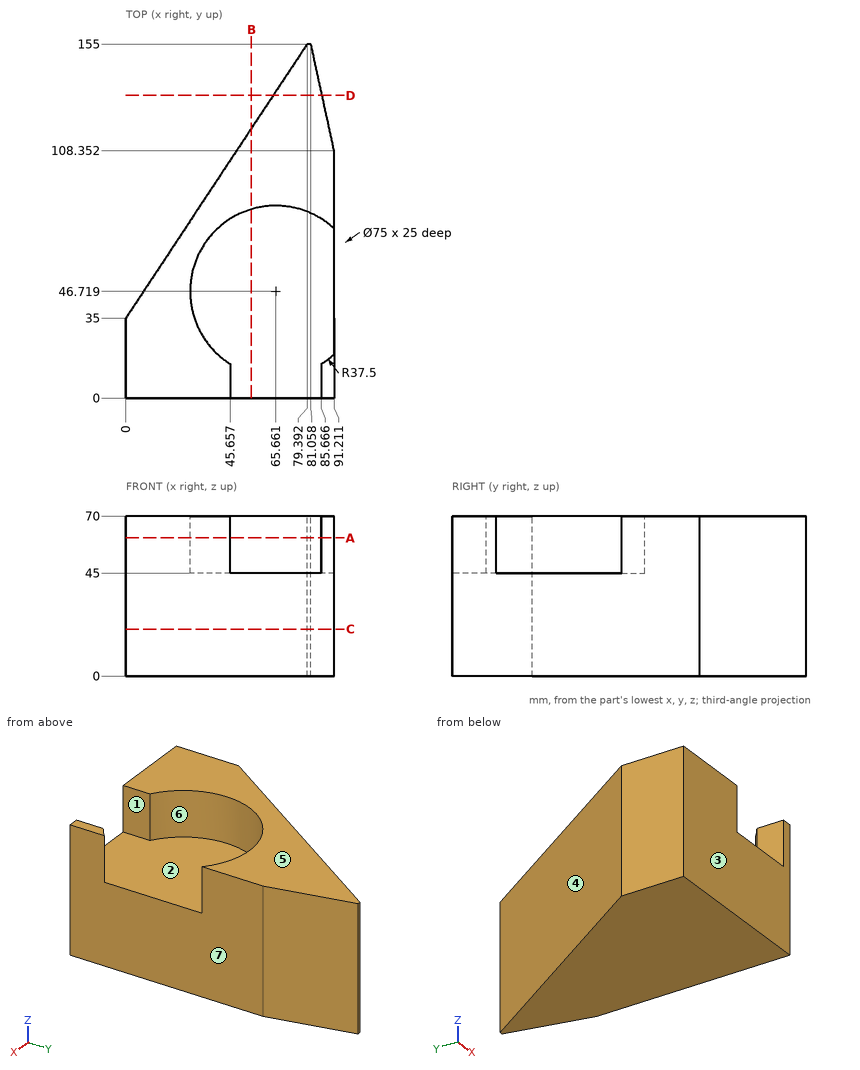
Input: dimensioned drawing with shaded views. Units: mm. Origin: part minimum x, y, z. A direction names the side the tool comes from. Coordinates: 2 decimals unless noted, no trailing zeros. Order: outer loops, then holes, each group sorted by start corner. A loop starts at its lowest first (then second) coordinate and runs counter-clockwise, first axis right, second up.
Item 1: Section query C-C (z = 20.5). Output: boundary loops of the cut face in (x, y).
Answer:
outline: (0, 0) - (91.21, 0) - (91.21, 108.35) - (81.06, 155) - (79.39, 155) - (0, 35) - close
Item 2: Access query for the marked faces 1, 2 and 3. Directions: +Z, -Z, +X, -X, +Y, -Y. A direction counts if a zero-diameter tool reaches every point of the face in a straight line with its end or side. Return the directions, or none.
Answer:
face 1: +Z, -Y
face 2: +Z
face 3: +Z, -Z, +X, -X, -Y
Item 3: Section query D-D (y = 132.5). Output: boundary loops of the cut face in (x, z) (1 decimal), then the cut area to 3 significant figures.
Answer:
outline: (64.5, 0) - (86, 0) - (86, 70) - (64.5, 70) - close
area: 1,500 mm2
Item 4: Draft query along X for the marked faces 4, 5, 6 and 7. Return one class per face: released by +X, released by -X, zero draft, split by the parting line, or undercut.
Answer:
face 4: released by -X
face 5: zero draft
face 6: undercut
face 7: released by +X
Item 5: Section query B-B (x = 55). Output: boundary loops of the cut face in (y, z), then the cut area to 3 significant figures.
Answer:
outline: (0, 0) - (118.13, 0) - (118.13, 70) - (82.67, 70) - (82.67, 45) - (0, 45) - close
area: 6,200 mm2
Item 6: Section query A-A (z = 60.5). Output: boundary loops of the cut face in (x, y) (1 decimal), then the cut area to 3 significant figures.
Answer:
outline: (0, 0) - (45.7, 0) - (45.7, 15) arc R37.5 cw (long way) to (91.2, 74.2) - (91.2, 108.4) - (81.1, 155) - (79.4, 155) - (0, 35) - close; (85.7, 0) - (91.2, 0) - (91.2, 19.3) arc R37.5 cw to (85.7, 15) - close
area: 4,730 mm2
Item 7: Material intervals for line 1 along X through (y, z) = (10, 47) (1 decimal); line 2 along Z through (x, y) = (30.5, 57); line 3 along Y through (x, z) = (41, 53) (1 decimal), sorted ascending.
Answer:
line 1: x = 0 to 45.7, 85.7 to 91.2
line 2: z = 0 to 45
line 3: y = 0 to 18.5, 75 to 97
Item 8: Contact query for flat-ended pins moving along their axis: P1, Ø1, axis at x = 9.5, z = 8, coming from the +Y side (1 decimal); P2, Ø4, axis at y = 137.5, z = 24.5, coming from the +X side; P3, Ø19, axis at x = 68, y = 35.5, coming from the +Z side. Output: stop coordinate, or through.
Answer:
P1: stops at y = 50.1
P2: stops at x = 85.3
P3: stops at z = 45
